Geometry check sheet. Reference: the model listing, model coordinates, mm. Face numbers are marked on the shaded views. A direction names the side the tool comes from. Round coordinates to 2 decimals unless told otherwise and drop trailing zeros. Write each loop counter-clockwise with the first axis right and the second up, starting at its lowest first coordinate (ties: lowest second). Pieces come first, ordered by that corner, then holes. Notation, with made-up numbers: (60, -18) - (69, -18) arc R16 cw to (69, 12) - close; hole circle Ø11 at (42.25, 39.25). An arc over 180 degrees is marked (long way). Return JSON: item names as keys, results as strings.
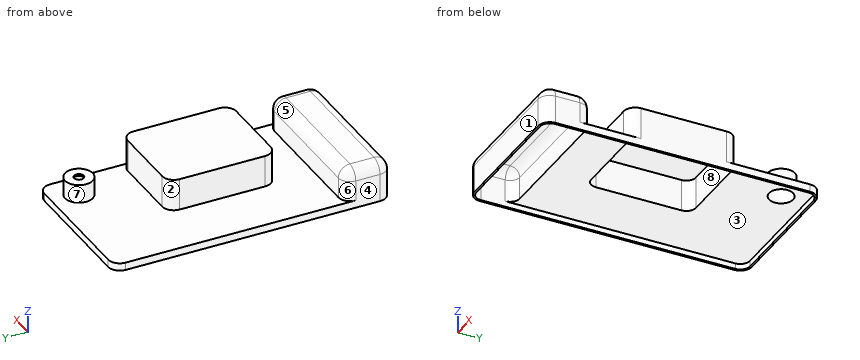
```python
from build123d import *

# Parameters (mm, degrees)
SKIZZE2_W                       = 144.44
SKIZZE2_H                       = 77
AUFSATZ_LINEAR_AUSTRAGEN1_DEPTH = 4
SKIZZE4_W                       = 77
SKIZZE4_H                       = 24.6
AUFSATZ_LINEAR_AUSTRAGEN2_DEPTH = 16.6
VERRUNDUNG2_R                   = 6
SKIZZE5_W                       = 47
SKIZZE5_H                       = 56.5
AUFSATZ_LINEAR_AUSTRAGEN3_DEPTH = 16.6
VERRUNDUNG4_R                   = 6
SKIZZE7_R                       = 7.25
AUFSATZ_LINEAR_AUSTRAGEN5_DEPTH = 9.6
VERRUNDUNG5_R                   = 6
VERRUNDUNG7_R                   = 6
WANDUNG2_T                      = -1
SKIZZE8_R                       = 2.5
SCHNITT_LINEAR_AUSTRAGEN1_DEPTH = 83.963476301


with BuildPart() as part:
    # Skizze2 → Aufsatz-Linear austragen1 (new body)
    with BuildSketch(Plane(origin=(0, 0, 0), x_dir=(0, 1, 0), z_dir=(0, 0, 1))):
        Rectangle(SKIZZE2_W, SKIZZE2_H)
    extrude(amount=AUFSATZ_LINEAR_AUSTRAGEN1_DEPTH)

    # Skizze4 → Aufsatz-Linear austragen2 (add)
    with BuildSketch(Plane.XY.offset(4)):
        with Locations((0, -59.92)):
            Rectangle(SKIZZE4_W, SKIZZE4_H)
    extrude(amount=AUFSATZ_LINEAR_AUSTRAGEN2_DEPTH)

    # Verrundung2
    verrundung2_edges = [part.edges().sort_by_distance(p)[0] for p in [
        (38.5, 72.22, 2),
        (38.5, -72.22, 10.3),
        (-38.5, -72.22, 10.3),
        (-38.5, 72.22, 2),
    ]]
    fillet(verrundung2_edges, radius=VERRUNDUNG2_R)

    # Skizze5 → Aufsatz-Linear austragen3 (add)
    with BuildSketch(Plane.XY.offset(4)):
        with Locations((15, 0.53)):
            Rectangle(SKIZZE5_W, SKIZZE5_H)
    extrude(amount=AUFSATZ_LINEAR_AUSTRAGEN3_DEPTH)

    # Verrundung4
    verrundung4_edges = [part.edges().sort_by_distance(p)[0] for p in [
        (38.5, -27.72, 12.3),
        (38.5, 28.78, 12.3),
        (-8.5, 28.78, 12.3),
        (-8.5, -27.72, 12.3),
    ]]
    fillet(verrundung4_edges, radius=VERRUNDUNG4_R)

    # Skizze7 → Aufsatz-Linear austragen5 (add)
    with BuildSketch(Plane.XY.offset(4)):
        with Locations(Location((24.503110224, 58.349132978, 0), (0, 0, 180))):
            Circle(SKIZZE7_R)
    extrude(amount=AUFSATZ_LINEAR_AUSTRAGEN5_DEPTH)

    # Verrundung5
    verrundung5_edges = [part.edges().sort_by_distance(p)[0] for p in [
        (0, -47.62, 20.6),
    ]]
    fillet(verrundung5_edges, radius=VERRUNDUNG5_R)

    # Verrundung7
    verrundung7_edges = [part.edges().sort_by_distance(p)[0] for p in [
        (-38.5, -59.92, 20.6),
        (-38.5, -47.62, 9.3),
        (-38.5, -49.377359313, 18.842640687),
        (38.5, -47.62, 9.3),
        (38.5, -49.377359313, 18.842640687),
        (38.5, -59.92, 20.6),
        (0, -72.22, 20.6),
        (-36.742640687, -70.462640687, 20.6),
        (36.742640687, -70.462640687, 20.6),
    ]]
    fillet(verrundung7_edges, radius=VERRUNDUNG7_R)

    # Wandung2
    wandung2_openings = [part.faces().sort_by_distance(p)[0] for p in [
        (0, 0, 0),
    ]]
    offset(amount=WANDUNG2_T, openings=wandung2_openings, kind=Kind.INTERSECTION)

    # Skizze8 → Schnitt-Linear austragen1 (cut, through all)
    with BuildSketch(Plane.XY.offset(13.6)):
        with Locations((24.503110224, 58.349132978)):
            Circle(SKIZZE8_R)
    extrude(amount=-SCHNITT_LINEAR_AUSTRAGEN1_DEPTH, mode=Mode.SUBTRACT)


solid = part.part
```
(1) Section check B-B, the plane x = 14.5. Enter the section's corners in (y, z), plus the area to 3 significant figures.
Response values:
{"outline": "(-72.22, 0) - (-71.22, 0) - (-71.22, 14.6) arc R5 cw to (-66.22, 19.6) - (-53.62, 19.6) arc R5 cw to (-48.62, 14.6) - (-48.62, 3) - (-26.72, 3) - (-26.72, 19.6) - (27.78, 19.6) - (27.78, 3) - (71.22, 3) - (71.22, 0) - (72.22, 0) - (72.22, 4) - (28.78, 4) - (28.78, 20.6) - (-27.72, 20.6) - (-27.72, 4) - (-47.62, 4) - (-47.62, 14.6) arc R6 ccw to (-53.62, 20.6) - (-66.22, 20.6) arc R6 ccw to (-72.22, 14.6) - close", "area": "212 mm^2"}
(2) Release check for a two-part mould opening along Y. For the marked faces 1, 2, 3 and 4 record: pulls with the +Y half, pulls with the -Y half, needs draft (parallel to the pull), parting line crosses it, or undercut.
Response values:
{"face 1": "pulls with the -Y half", "face 2": "pulls with the +Y half", "face 3": "undercut", "face 4": "needs draft"}
(3) Gauge pin test, flat ends, axial feed: pin 1 (6.5 mm diameter, centred on x = 24.5, y = 58.35, fed in from +Z); pin 2 (1 mm diameter, centred on x = 11, y = 1, fed in from -Z); pin 3 (8.5 mm diameter, centred on x = 7.5, z = 11.5, fed in from +Y). Record the tip position at first contact, or that the pin passes through.
Response values:
{"pin 1": "stops at z = 13.6", "pin 2": "stops at z = 19.6", "pin 3": "stops at y = 28.78"}
(4) Section check A-A, the plane z = 16. Give the number of separate pieces and of enclosed holes in the cut face, plus the area to 3 significant figures.
Response values:
{"separate pieces": "2", "enclosed holes": "2", "area": "389 mm^2"}
(5) Access from +Z, -Z, +X, -X, +Y, -Y to the whole of each face (thin tool, end or side, straight path). Record for the marked faces 5, 6, 7 and 8.
Response values:
{"face 5": "+Z, +X, -X", "face 6": "+Z, -X, +Y", "face 7": "+Z", "face 8": "-Z"}
(6) Material ranges on line 1 along Y through (x, z) = (17, 9.75); line 2 along Y through (x, z) = (-31, 2); line 3 along Y through (x, z) = (-9, 13), recorded low to high. Write a range as [from, to].
Response values:
{"line 1": "y = [-72.22, -71.22], [-48.62, -47.62], [-27.72, -26.72], [27.78, 28.78]", "line 2": "y = [-72.22, -71.22], [71.22, 72.22]", "line 3": "y = [-72.22, -71.22], [-48.62, -47.62]"}
(7) Section check D-D, the plane y = 16. Enter the section's corners in (x, z), plus the area to 3 significant figures.
Response values:
{"outline": "(-38.5, 0) - (-37.5, 0) - (-37.5, 3) - (-7.5, 3) - (-7.5, 19.6) - (37.5, 19.6) - (37.5, 0) - (38.5, 0) - (38.5, 20.6) - (-8.5, 20.6) - (-8.5, 4) - (-38.5, 4) - close", "area": "116 mm^2"}
(8) Section check C-C, the plane z = 1.5. Enter the section's corners in (x, y), plus the area to 3 significant figures.
Response values:
{"outline": "(-38.5, -66.22) arc R6 ccw to (-32.5, -72.22) - (32.5, -72.22) arc R6 ccw to (38.5, -66.22) - (38.5, 66.22) arc R6 ccw to (32.5, 72.22) - (-32.5, 72.22) arc R6 ccw to (-38.5, 66.22) - close; hole (-37.5, -66.22) arc R5 ccw to (-32.5, -71.22) - (32.5, -71.22) arc R5 ccw to (37.5, -66.22) - (37.5, 66.22) arc R5 ccw to (32.5, 71.22) - (-32.5, 71.22) arc R5 ccw to (-37.5, 66.22) - close", "area": "429 mm^2"}
